Read the model definition and answer for the solid it produces. Units are mm, in the model's axes. A direction names the side the tool comes from. Coordinates: 2 decimals unless noted, no trailing zeros. Write each loop counter-clockwise with the first axis right and the second up, starting at its lowest first coordinate (ties: lowest second). Pieces come first, ordered by that corner, then holes. Notation, with made-up numbers: (-25, -32.5) -> (-1, -32.5) arc R25 cw to (-1, -4.5) -> close; hole circle Ø10 at (61.5, -34). An arc over 180 degrees is marked (long way). Answer in a Markdown table with one row per item. Add a question column.
Item 1: Given pin 1 Ø1.5 at (x, z) = (4, 1) entering from +Y, flat-ended and moving along its own axis, determine where the tip first touches the part or whether it passes through.
Item 2: Section B-B on y = 20 is taken. Write down the section's boundary in (x, z).
Item 3: Which of the six approach directions +Z, -Z, +X, -X, +Y, -Y give full straight-line access (tool end or side, diameter ignored) to faces 1 (the face through (0, 0, 0)), 2 (the face through (-0.27, 18.54, 1.22))?
Item 4: Section C-C on z = 3.75 is taken. Write down the section's boundary in (x, y).
Item 5: Section D-D on z = -4 is taken. Write down the section's boundary in (x, y).
Item 6: Section A-A on x = 0 is taken. Write down the section's boundary in (y, z).
Item 7: Straight lines are drawn through the part: line 1 (Y direction, x = 5.75, z = 5); line 2 (X direction, y = 3, z = -3.5); line 3 (Z direction, x = -6.5, y = 2.5). For each, find the intervals that lie inside material, in ascending order. Write a range as from..to.
```python
from build123d import *

# Parameters (mm, degrees)
BOSS_EXTRUDE1_DEPTH = 3.75
SKETCH4_R           = 1.25
BOSS_EXTRUDE2_DEPTH = 30


with BuildPart() as part:
    # Sketch1 → Boss-Extrude1 (new body)
    with BuildSketch(Plane(origin=(0, 0, 0), x_dir=(1, 0, 0), z_dir=(0, 1, 0))):
        Polygon((9.237604307, 0), (4.618802154, 8), (-4.618802154, 8), (-9.237604307, 0), (-4.618802154, -8), (4.618802154, -8), align=None)
    extrude(amount=BOSS_EXTRUDE1_DEPTH)

    # Sketch2 → Cut-Revolve1 (revolve, cut)
    with BuildSketch(Plane.XY):
        with BuildLine():
            Line((9.237604307, 2.75), (9.237604307, 3.75))
            Line((9.237604307, 3.75), (8.237604307, 3.75))
            ThreePointArc((8.237604307, 3.75), (8.944711088, 3.457106781), (9.237604307, 2.75))
        make_face()
    revolve(axis=Axis((0, 0, 0), (0, 1, 0)), mode=Mode.SUBTRACT)

    # Sketch3 → Cut-Revolve2 (revolve, cut)
    with BuildSketch(Plane.XY):
        with BuildLine():
            Line((9.237604307, 0), (8.237604307, 0))
            ThreePointArc((8.237604307, 0), (8.944711088, 0.292893219), (9.237604307, 1))
            Line((9.237604307, 1), (9.237604307, 0))
        make_face()
    revolve(axis=Axis((0, 0, 0), (0, 1, 0)), mode=Mode.SUBTRACT)

    # Sketch4 → Boss-Extrude2 (add)
    with BuildSketch(Plane(origin=(0, 3.75, 0), x_dir=(1, 0, 0), z_dir=(0, 1, 0))):
        Circle(SKETCH4_R)
    extrude(amount=BOSS_EXTRUDE2_DEPTH)


solid = part.part
```
Results below:
| question | item | result |
|---|---|---|
| 1 | pin 1 | stops at y = 3.75 |
| 2 | outline | circle Ø2.5 at (0, 0) |
| 3 | face 1 | +Z, -Z, +X, -X, -Y |
| 3 | face 2 | +Y |
| 4 | outline | (-7.07, 0) -> (7.07, 0) -> (7.07, 3.75) -> (-7.07, 3.75) -> close |
| 5 | outline | (-6.93, 0) -> (6.93, 0) -> (6.93, 3.75) -> (-6.93, 3.75) -> close |
| 6 | outline | (0, -8) -> (3.75, -8) -> (3.75, -1.25) -> (33.75, -1.25) -> (33.75, 1.25) -> (3.75, 1.25) -> (3.75, 8) -> (0, 8) -> close |
| 7 | line 1 | y = 0..3.75 |
| 7 | line 2 | x = -7.22..7.22 |
| 7 | line 3 | z = -4.74..4.74 |
